Answer from the drawing. Dimensions are ordinates in mm from the lowest x, y and z of the part. A direction names the side the tool comes from. Coordinates: 2 decimals unless noted, no trailing zeros. Order: outer loops, then holes, each group sorted by start corner. A loop starts at its lowest first (then second) coordinate and runs counter-clockwise, first axis right, second up.
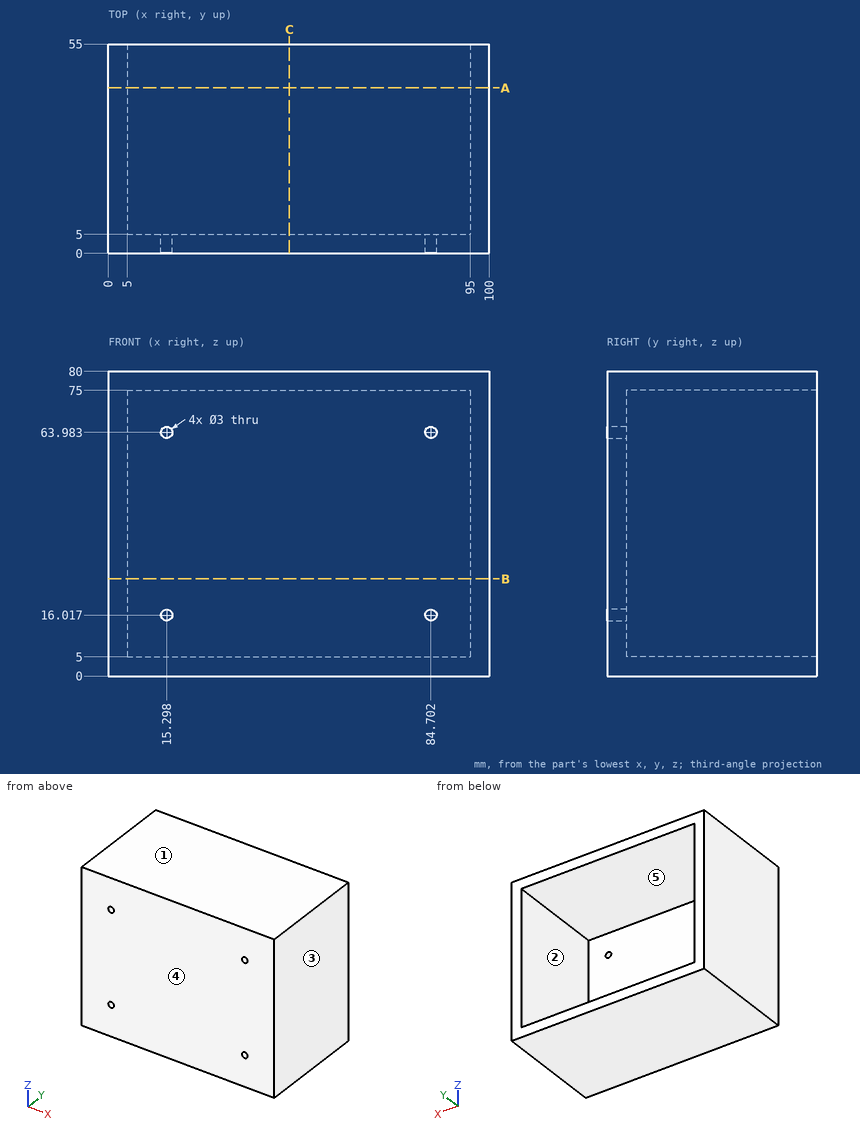
1. The mould has two halves that part along Z. Classify the marked faces 1, 2 and 3: released by +Z, released by -Z, zero draft, split by the parting line, or undercut.
2. Flat-ended cylindrical pins translate along their axes: pin 1 (1.8 mm diameter, centred on x = 84.7, z = 16.02, fed in from +Y); pin 2 (2 mm diameter, centred on x = 57, z = 39.5, fed in from +Y). Find the tip coordinate at first contact, or state that the pin passes through.
3. The part is cut by section A-A (y = 43.5). Determine the outline of the cut face in (x, z).
4. The part is cut by section B-B (z = 25.5). Determine the outline of the cut face in (x, y), plus the area to 3 significant figures.
5. Consider probe 1 along Z at (x, y) = (70, 5.5); probe 2 along X at (y, z) = (26, 37); probe 3 along Y at (x, z) = (70, 45). Determine where each line is inside the solid, lowest interval first.
6. The part is cut by section C-C (x = 47.5). Determine the outline of the cut face in (y, z).
7. For the marked faces 4 and 5, determine the directions among +Z, -Z, +X, -X, +Y, -Y from which every point of the face is accessible in a straight line to the end or side of a thin tool.
Worked out:
1. face 1: released by +Z
1. face 2: undercut
1. face 3: zero draft
2. pin 1: passes through
2. pin 2: stops at y = 5
3. outline: (0, 0) - (100, 0) - (100, 80) - (0, 80) - close; hole (5, 5) - (95, 5) - (95, 75) - (5, 75) - close
4. outline: (0, 0) - (100, 0) - (100, 55) - (95, 55) - (95, 5) - (5, 5) - (5, 55) - (0, 55) - close
4. area: 1,000 mm2
5. probe 1: z = 0 to 5, 75 to 80
5. probe 2: x = 0 to 5, 95 to 100
5. probe 3: y = 0 to 5
6. outline: (0, 0) - (55, 0) - (55, 5) - (5, 5) - (5, 75) - (55, 75) - (55, 80) - (0, 80) - close
7. face 4: +Z, -Z, +X, -X, -Y
7. face 5: +Y
